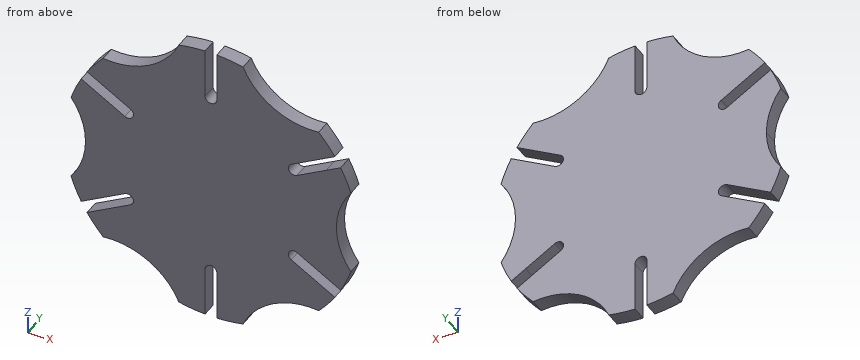
```python
from build123d import *

# Parameters (mm, degrees)
BOSS_EXTRUDE1_DEPTH = 5


with BuildPart() as part:
    # Sketch1 → Boss-Extrude1 (new body)
    with BuildSketch(Plane(origin=(0, 0, 0), x_dir=(1, 0, 0), z_dir=(0, 1, 0))):
        with BuildLine():
            ThreePointArc((47.726299074, 14.90638711), (46.185164881, 19.155431211), (44.266615306, 23.247941186))
            Line((44.266615306, 23.247941186), (39.371782551, 20.421908177))
            ThreePointArc((39.371782551, 20.421908177), (32.796167617, 0), (39.371782551, -20.421908177))
            Line((39.371782551, -20.421908177), (44.266615306, -23.247941186))
            ThreePointArc((44.266615306, -23.247941186), (46.185164881, -19.155431211), (47.726299074, -14.90638711))
            ThreePointArc((47.726299074, -14.90638711), (42.796167617, 0), (47.726299074, 14.90638711))
        make_face()
        with BuildLine():
            ThreePointArc((39.371782551, -20.421908177), (32.796167617, 0), (39.371782551, 20.421908177))
            Line((39.371782551, 20.421908177), (29.402314303, 14.666033001))
            ThreePointArc((29.402314303, 14.666033001), (26.670263496, 15.398083809), (27.402314303, 18.130134616))
            Line((27.402314303, 18.130134616), (42.266615306, 26.712042801))
            ThreePointArc((42.266615306, 26.712042801), (39.68167249, 30.41981046), (36.772459453, 33.878993872))
            ThreePointArc((36.772459453, 33.878993872), (21.398083809, 37.062568341), (10.953839621, 48.785380982))
            ThreePointArc((10.953839621, 48.785380982), (6.503492392, 49.575241671), (2, 49.959983987))
            Line((2, 49.959983987), (2, 32.796167617))
            ThreePointArc((2, 32.796167617), (0, 30.796167617), (-2, 32.796167617))
            Line((-2, 32.796167617), (-2, 49.959983987))
            ThreePointArc((-2, 49.959983987), (-6.503492392, 49.575241671), (-10.953839621, 48.785380982))
            ThreePointArc((-10.953839621, 48.785380982), (-21.398083809, 37.062568341), (-36.772459453, 33.878993872))
            ThreePointArc((-36.772459453, 33.878993872), (-39.68167249, 30.41981046), (-42.266615306, 26.712042801))
            Line((-42.266615306, 26.712042801), (-27.402314303, 18.130134616))
            ThreePointArc((-27.402314303, 18.130134616), (-26.670263496, 15.398083809), (-29.402314303, 14.666033001))
            Line((-29.402314303, 14.666033001), (-44.266615306, 23.247941186))
            ThreePointArc((-44.266615306, 23.247941186), (-46.185164881, 19.155431211), (-47.726299074, 14.90638711))
            ThreePointArc((-47.726299074, 14.90638711), (-44.060680329, 7.850263895), (-42.796167617, 0))
            ThreePointArc((-42.796167617, 0), (-44.060680329, -7.850263895), (-47.726299074, -14.90638711))
            ThreePointArc((-47.726299074, -14.90638711), (-46.185164881, -19.155431211), (-44.266615306, -23.247941186))
            Line((-44.266615306, -23.247941186), (-29.402314303, -14.666033001))
            ThreePointArc((-29.402314303, -14.666033001), (-26.670263496, -15.398083809), (-27.402314303, -18.130134616))
            Line((-27.402314303, -18.130134616), (-42.266615306, -26.712042801))
            ThreePointArc((-42.266615306, -26.712042801), (-39.68167249, -30.41981046), (-36.772459453, -33.878993872))
            ThreePointArc((-36.772459453, -33.878993872), (-21.398083809, -37.062568341), (-10.953839621, -48.785380982))
            ThreePointArc((-10.953839621, -48.785380982), (-6.503492392, -49.575241671), (-2, -49.959983987))
            Line((-2, -49.959983987), (-2, -32.796167617))
            ThreePointArc((-2, -32.796167617), (0, -30.796167617), (2, -32.796167617))
            Line((2, -32.796167617), (2, -49.959983987))
            ThreePointArc((2, -49.959983987), (6.503492392, -49.575241671), (10.953839621, -48.785380982))
            ThreePointArc((10.953839621, -48.785380982), (21.398083809, -37.062568341), (36.772459453, -33.878993872))
            ThreePointArc((36.772459453, -33.878993872), (39.68167249, -30.41981046), (42.266615306, -26.712042801))
            Line((42.266615306, -26.712042801), (27.402314303, -18.130134616))
            ThreePointArc((27.402314303, -18.130134616), (26.670263496, -15.398083809), (29.402314303, -14.666033001))
            Line((29.402314303, -14.666033001), (39.371782551, -20.421908177))
        make_face()
    extrude(amount=BOSS_EXTRUDE1_DEPTH)


solid = part.part
```
Geometry: final body of the model. Coordinates: model frame, mm. Round coordinates to 2 decimals unless told otherwise and drop trailing zeros. Order: outer loops, then holes, each group sorted by start corner. A loop starts at its lowest first (then second) coordinate and runs counter-clockwise, first axis right, second up. Notation, with made-up numbers: (76, -24.75) - (101, -24.75) arc R24 cw to (101, 3.25) - close; hole circle Ø7 at (0.5, 15). An arc over 180 degrees is marked (long way). Write item = value, one per line. Start each with the question number.
Q1. Ray query, line 1 (Z direction, x = -28, y = 3.35); line 2 (X direction, y = 4.6, z = 16.5); line 3 (Z direction, x = -30, y = 4.8). Return the intervals inside material, ascending. Write a range as from..to.
Q2. Cut plane B-B on x = 0. Return the cut outline in (y, z).
Q3. Cut plane D-D on z = -10.5. Return the cut outline in (x, y), and give its area (3 significant figures).
Q4. Pin query (flat end, axial travel): pin 1 (3 mm diameter, centred on x = -20.5, y = 3, fed in from +Z); pin 2 (1.5 mm diameter, centred on x = 22.5, y = 3.5, fed in from +Z); pin 3 (2 mm diameter, centred on x = -11, y = 2.5, fed in from +Z). Return the tip coordinate at first contact, or that it passes through.
Q5. Cut plane A-A on z = -43. Return the cut outline in (x, y).
Q6. Cut plane C-C on z = 37. Return the cut outline in (x, y).
Outcome:
q1.line_1 = -34.42..-18.48, -14.44..14.44, 18.48..34.42
q1.line_2 = -47.2..-32.58, -26.4..26.4, 32.58..47.2
q1.line_3 = -34.02..-19.63, -15.01..15.01, 19.63..34.02
q2.outline = (0, -30.8) - (5, -30.8) - (5, 30.8) - (0, 30.8) - close
q3.outline = (-45.11, 0) - (45.11, 0) - (45.11, 5) - (-45.11, 5) - close
q3.area = 451 mm^2
q4.pin_1 = 38.64
q4.pin_2 = 36.86
q4.pin_3 = 48.99
q5.outline = (-14.45, 0) - (-2, 0) - (-2, 5) - (-14.45, 5) - close; (2, 0) - (14.45, 0) - (14.45, 5) - (2, 5) - close
q6.outline = (-21.51, 0) - (-2, 0) - (-2, 5) - (-21.51, 5) - close; (2, 0) - (21.51, 0) - (21.51, 5) - (2, 5) - close
